For this review, use the dimensioned drawing (mm, ordinates from the lowest corner) and the shaded views. Coordinates: 2 decimals unless noted, no trailing zeros. Loops run counter-clockwise (first coordinate to the right, second up) from the corner with the lowest first, then second, coordinate; pieces in that order, holes last. Notation, with made-up numbers: (67.25, 81.25) - (125.25, 81.25) arc R5 ccw to (125.25, 88.25) - close; hole circle Ø5 at (86.25, -7). An arc over 180 degrees is marked (long way). Answer in a Markdown table with one row per item. Add a question column.
(1) We need section B-B, the plane z = 6. Write out the cut boundary in (x, y), plus the area to 3 significant figures.
(2) Clearance check with flat-ended pins moving along their axes: pin 1 (0.5 mm diameter, centred on x = 2.5, y = 2.5, fed in from -Z); pin 2 (1 mm diameter, centred on y = 2.5, z = 5, fed in from -X). State where each tip first meets the part, or that it passes through.
(3) We need section D-D, the plane y = 2.7. Write out the cut boundary in (x, z).
(4) We need section C-C, the plane x = 1.4. Write out the cut boundary in (y, z).
(5) To check wall thickness, follow L1, parallel to X at y = 2.15, z = 4.75; L2, parallel to Z at x = 2.9, y = 2.8; L3, parallel to Z at x = 4.45, y = 2.9. State the ranges of each line that lie inside material, in increasing order. Write a range as [from, to].
(6) We need section A-A, the plane y = 2. Write out the cut boundary in (x, z).
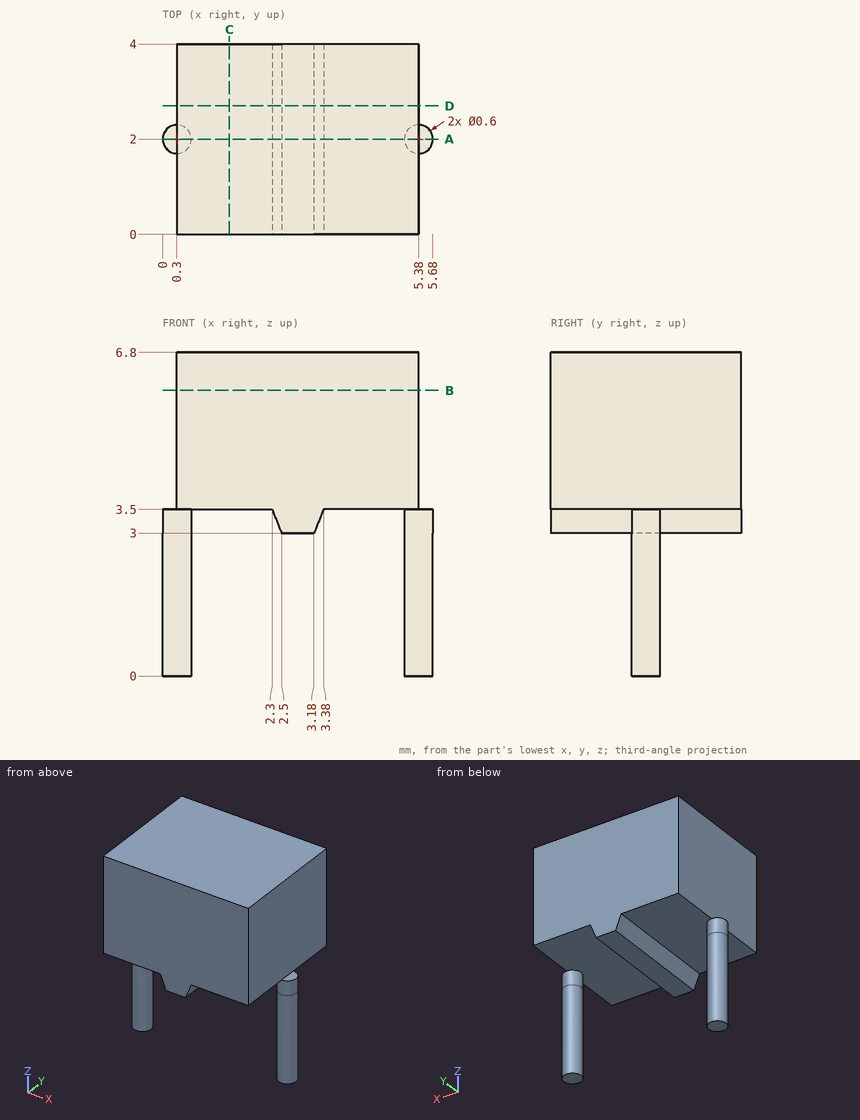
Responses:
| question | item | result |
|---|---|---|
| 1 | outline | (0.3, 0) - (5.38, 0) - (5.38, 4) - (0.3, 4) - close |
| 1 | area | 20.3 mm2 |
| 2 | pin 1 | stops at z = 3 |
| 2 | pin 2 | stops at x = 0.3 |
| 3 | outline | (0.3, 3.5) - (2.3, 3.5) - (2.5, 3) - (3.18, 3) - (3.38, 3.5) - (5.38, 3.5) - (5.38, 6.8) - (0.3, 6.8) - close |
| 4 | outline | (0, 3.5) - (4, 3.5) - (4, 6.8) - (0, 6.8) - close |
| 5 | L1 | x = [0.3, 5.38] |
| 5 | L2 | z = [3, 6.8] |
| 5 | L3 | z = [3.5, 6.8] |
| 6 | outline | (0, 0) - (0.6, 0) - (0.6, 3.5) - (2.3, 3.5) - (2.5, 3) - (3.18, 3) - (3.38, 3.5) - (5.08, 3.5) - (5.08, 0) - (5.68, 0) - (5.68, 3.5) - (5.38, 3.5) - (5.38, 6.8) - (0.3, 6.8) - (0.3, 3.5) - (0, 3.5) - close |
